Design review of the part built by this model. Coordinates are the model's own, in mm. Face numbers are marked on the shaded views. A direction names the side the tool comes from. Coordinates: 2 decimals unless noted, no trailing zeros. Loops run counter-clockwise (first coordinate to the right, second up) from the corner with the lowest first, then second, coordinate; pieces in that order, holes last. Notation, with made-up numbers: M -22,-37.75 L 8,-37.75 A25 ccw 8,-6.75 Z; hole C 3,8 d1. An arc over 180 degrees is marked long. One line per item, written item: value.
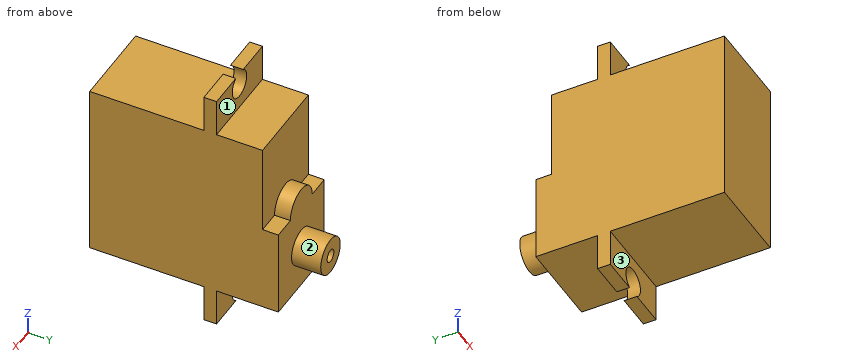
```python
from build123d import *

# Parameters (mm, degrees)
SKETCH1_W           = 13.6
SKETCH1_H           = 28.4
BOSS_EXTRUDE1_DEPTH = 27.25
BOSS_EXTRUDE2_DEPTH = 2.5
SKETCH3_R           = 2.9
SKETCH3_R_2         = 1
BOSS_EXTRUDE3_DEPTH = 4.6
SKETCH5_W           = 13.6
SKETCH5_H           = 40.4
BOSS_EXTRUDE5_DEPTH = 2
SKETCH8_R           = 2.15
CUT_EXTRUDE1_DEPTH  = 2
SKETCH7_R           = 2.15
CUT_EXTRUDE2_DEPTH  = 2


with BuildPart() as part:
    # Sketch1 → Boss-Extrude1 (new body)
    with BuildSketch(Plane(origin=(0, 0, 0), x_dir=(1, 0, 0), z_dir=(0, 1, 0))):
        Rectangle(SKETCH1_W, SKETCH1_H)
    extrude(amount=BOSS_EXTRUDE1_DEPTH)

    # Sketch2 → Boss-Extrude2 (add)
    with BuildSketch(Plane(origin=(0, 27.25, 0), x_dir=(1, 0, 0), z_dir=(0, 1, 0))):
        with BuildLine():
            ThreePointArc((-3.25, 0.2), (0, -3.05), (3.25, 0.2))
            Line((3.25, 0.2), (-3.25, 0.2))
        make_face()
        with BuildLine():
            Line((-3.25, 0.2), (3.25, 0.2))
            ThreePointArc((3.25, 0.2), (0, 3.45), (-3.25, 0.2))
        make_face()
        with BuildLine():
            Line((6.8, 0.2), (6.8, 14.2))
            Line((6.8, 14.2), (-6.8, 14.2))
            Line((-6.8, 14.2), (-6.8, 0.2))
            Line((-6.8, 0.2), (-3.25, 0.2))
            ThreePointArc((-3.25, 0.2), (0, 3.45), (3.25, 0.2))
            Line((3.25, 0.2), (6.8, 0.2))
        make_face()
    extrude(amount=BOSS_EXTRUDE2_DEPTH)

    # Sketch3 → Boss-Extrude3 (add)
    with BuildSketch(Plane(origin=(0, 29.75, 0), x_dir=(1, 0, 0), z_dir=(0, 1, 0))):
        with Locations(Location((0, 7.2, 0), (0, 0, 270))):
            Circle(SKETCH3_R)
        with Locations(Location((0, 7.2, 0), (0, 0, 270))):
            Circle(SKETCH3_R_2, mode=Mode.SUBTRACT)
    extrude(amount=BOSS_EXTRUDE3_DEPTH)

    # Sketch5 → Boss-Extrude5 (add)
    with BuildSketch(Plane(origin=(0, 20, 0), x_dir=(-1, 0, 0), z_dir=(0, -1, 0))):
        Rectangle(SKETCH5_W, SKETCH5_H)
    extrude(amount=BOSS_EXTRUDE5_DEPTH)

    # Sketch8 → Cut-Extrude1 (cut)
    with BuildSketch(Plane(origin=(0, 20, 0), x_dir=(1, 0, 0), z_dir=(0, 1, 0))):
        with Locations((0, -18.35)):
            Circle(SKETCH8_R)
    extrude(amount=-CUT_EXTRUDE1_DEPTH, mode=Mode.SUBTRACT)

    # Sketch7 → Cut-Extrude2 (cut)
    with BuildSketch(Plane(origin=(0, 20, 0), x_dir=(1, 0, 0), z_dir=(0, 1, 0))):
        with Locations((0, 18.35)):
            Circle(SKETCH7_R)
    extrude(amount=-CUT_EXTRUDE2_DEPTH, mode=Mode.SUBTRACT)


solid = part.part
```
(1) We need section A-A on z = -18.35. State the section outline as (x, y) points, then the cut area to 3 significant figures.
Reply:
outline: M -6.8,18 L -2.15,18 L -2.15,20 L -6.8,20 Z; M 2.15,18 L 6.8,18 L 6.8,20 L 2.15,20 Z
area: 18.6 mm2
(2) Insertion check: pin 1 (3 mm diameter, centred on x = -3, z = -16, fed in from -Y); pin 2 (2.5 mm diameter, centred on x = 0, z = -7.2, fed in from -Y); pin 3 (2 mm diameter, centred on x = 5, y = 28, fed in from +Z); pin 4 (1.5 mm diameter, centred on x = 4.5, z = -6, fed in from +Y). Each pin has a flat end and moves straight along its axis. Give the tip position at first contact, or say it passes through.
Reply:
pin 1: stops at y = 18
pin 2: stops at y = 0
pin 3: stops at z = 14.2
pin 4: stops at y = 29.75
(3) Tool access review of the marked faces 1, 2 and 3: name each direction out of +Z, -Z, +X, -X, +Y, -Y from which nothing blocks a thin tool from reaching the whole face with its end or side.
Reply:
face 1: +Z, +X, -X, +Y
face 2: +Y
face 3: -Z, +X, -X, -Y
(4) We need section C-C on z = -7.2. State the section outline as (x, y) points, then the cut area to 3 significant figures.
Reply:
outline: M -6.8,0 L 6.8,0 L 6.8,29.75 L 2.9,29.75 L 2.9,34.35 L 1,34.35 L 1,29.75 L -1,29.75 L -1,34.35 L -2.9,34.35 L -2.9,29.75 L -6.8,29.75 Z
area: 422 mm2
(5) We need section D-D on y = 32. State the section outline as (x, z) points, then the cut area to 3 significant figures.
Reply:
outline: C 0,-7.2 d5.8; hole C 0,-7.2 d2
area: 23.3 mm2
(6) We need section B-B on x = -4.5. State the section outline as (y, z) points.
Reply:
outline: M 0,-14.2 L 18,-14.2 L 18,-20.2 L 20,-20.2 L 20,-14.2 L 29.75,-14.2 L 29.75,-0.2 L 27.25,-0.2 L 27.25,14.2 L 20,14.2 L 20,20.2 L 18,20.2 L 18,14.2 L 0,14.2 Z
(7) To check wall thickness, follow line 1 along X through (y, z) = (19.3, 18.35); line 2 along Y through (x, z) = (-6, -4); line 3 along X through (y, z) = (32.1, -7.2). State the ranges of each line that lie inside material, in increasing order. Write a range as [from, to].
Reply:
line 1: x = [-6.8, -2.15], [2.15, 6.8]
line 2: y = [0, 29.75]
line 3: x = [-2.9, -1], [1, 2.9]
